For this review, take the finished solid that the model builds, in its own axes (mm). Face numbers are marked on the shaded views. A direction names the side the tool comes from. Give positions to 0.01 mm unless a question says otherwise; leave off trailing zeros. Write each loop counter-clockwise with the first axis right and the second up, starting at its lowest first coordinate (ties: lowest second). Pieces come first, ordered by that corner, then holes.
Q1. Machinability: for the marked faces 1 and 2, which of the approach directions +Z, -Z, +X, -X, +Y, -Y give a long, thin tool a straight path to every point of the face, cutting with its end or side? Answer none if there is none.
Q2. We need section B-B (z = 0.9). Write out the cut boundary in (x, y) (1 decimal).
Q3. For line 1 (X direction, y = -11, z = 0.2); line 2 (X direction, y = -11.5, z = 2.5); line 3 (Y direction, x = -11, z = 0.3), list the stretches that pass through material, from the lowest coordinate up.
Q4. We need section C-C (x = 4). Write out the cut boundary in (y, z) (1 decimal), then the cut area to 3 significant figures.
Q5. Mouldability with a two-part tool opening along X and no side actions: class the marked faces 3, 4, 5 and 6 as released by +X, released by -X, zero draft, split by the parting line, or undercut.
Q6. We need section D-D (y = -16). Write out the cut boundary in (x, z) (3 decimals), then the cut area to 3 significant figures.
Q7. Insertion check: P1, Ø3, axis at x = 7, y = -11.5, coming from the -Z side; P2, Ø1, axis at x = 2, z = 2.5, coming from the -Y side; P3, Ø1.6, axis at x = 4.5, z = 1, coming from the -Y side; P4, Ø1.5, axis at y = -15, z = 1.5, coming from the -X side. Each pin has a flat end and moves straight along its axis. Give the tip position at first contact, or say it passes through.
Q8. We need section A-A (x = -9.5). Write out the cut boundary in (y, z) (1 decimal), then the cut area to 3 significant figures.
```python
from build123d import *

# Parameters (mm, degrees)
BOSS_EXTRUDE1_DEPTH = 3.175
FILLET1_R           = 0.4
FILLET2_R           = 0.6


with BuildPart() as part:
    # Sketch1 → Boss-Extrude1 (new body)
    with BuildSketch(Plane.XY):
        with BuildLine():
            Line((-20.955, 0), (14.605, 0))
            ThreePointArc((14.605, 0), (-3.175, -17.78), (-20.955, 0))
        make_face()
        with BuildLine():
            Line((1.774264706, -4.7625), (8.940027858, -4.7625))
            ThreePointArc((8.940027858, -4.7625), (5.197167803, -9.968054601), (-0.576629116, -12.755538993))
            Line((-0.576629116, -12.755538993), (1.774264706, -4.7625))
        make_face(mode=Mode.SUBTRACT)
        with BuildLine():
            Line((-15.290027858, -4.7625), (-8.124264706, -4.7625))
            Line((-8.124264706, -4.7625), (-5.773370884, -12.755538993))
            ThreePointArc((-5.773370884, -12.755538993), (-11.547167803, -9.968054601), (-15.290027858, -4.7625))
        make_face(mode=Mode.SUBTRACT)
    extrude(amount=BOSS_EXTRUDE1_DEPTH)

    # Fillet1
    fillet1_edges = [part.edges().sort_by_distance(p)[0] for p in [
        (-5.773370884, -12.755538993, 1.5875),
        (-0.576629116, -12.755538993, 1.5875),
        (8.940027858, -4.7625, 1.5875),
        (-15.290027858, -4.7625, 1.5875),
    ]]
    fillet(fillet1_edges, radius=FILLET1_R)

    # Fillet2
    fillet2_edges = [part.edges().sort_by_distance(p)[0] for p in [
        (-8.124264706, -4.7625, 1.5875),
        (1.774264706, -4.7625, 1.5875),
    ]]
    fillet(fillet2_edges, radius=FILLET2_R)


solid = part.part
```
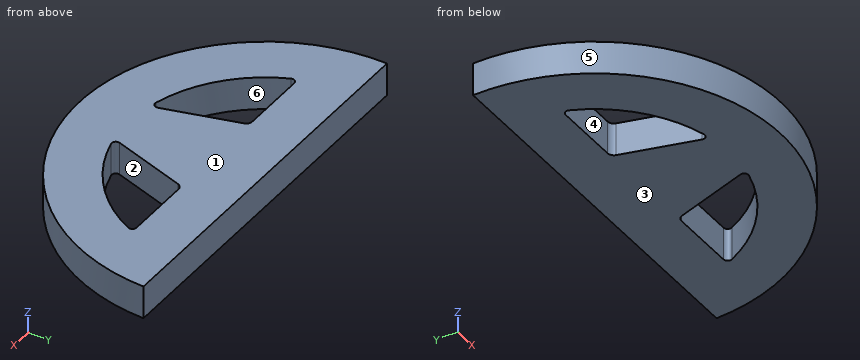
Computed:
1. face 1: +Z, +X, -X, +Y, -Y
1. face 2: +Z, -Z
2. outline: (-21, 0) arc R17.8 ccw to (14.6, 0) - close; hole (-15.1, -5.3) arc R13 ccw to (-6.5, -12.6) arc R0.4 ccw to (-6, -12.1) - (-8, -5.2) arc R0.6 ccw to (-8.6, -4.8) - (-14.7, -4.8) arc R0.4 ccw to start; hole (-0.4, -12.1) arc R0.4 ccw to (0.1, -12.6) arc R13 ccw to (8.7, -5.3) arc R0.4 ccw to (8.3, -4.8) - (2.2, -4.8) arc R0.6 ccw to (1.6, -5.2) - close
3. line 1: x = -17.14 to -10.14, -6.29 to -0.06, 3.79 to 10.79
3. line 2: x = -16.74 to -9.27, -6.14 to -0.21, 2.92 to 10.39
3. line 3: y = -15.97 to -10.4, -4.76 to 0
4. outline: (-16.3, 0) - (-10.9, 0) - (-10.9, 3.2) - (-16.3, 3.2) - close; (-4.8, 0) - (0, 0) - (0, 3.2) - (-4.8, 3.2) - close
4. area: 32.3 mm2
5. face 3: zero draft
5. face 4: undercut
5. face 5: split by the parting line
5. face 6: undercut
6. outline: (-10.929, 0) - (4.579, 0) - (4.579, 3.175) - (-10.929, 3.175) - close
6. area: 49.2 mm2
7. P1: stops at z = 0
7. P2: stops at y = -17.15
7. P3: stops at y = -16.4
7. P4: stops at x = -13.81
8. outline: (-16.6, 0) - (-11.4, 0) - (-11.4, 3.2) - (-16.6, 3.2) - close; (-4.8, 0) - (0, 0) - (0, 3.2) - (-4.8, 3.2) - close
8. area: 31.8 mm2
